For this review, take the finished solid that the model builds, in its own axes (mm). A direction names the side the tool comes from. Coordinates: 2 decimals unless noted, no trailing zeros. Loops run counter-clockwise (first coordinate to the right, second up) from the corner with the lowest first, then second, coordinate; pieces in that order, holes last. Notation, with made-up numbers: M 85,75.5 L 99,75.5 A28 cw 99,94.5 Z; hole C -39,-10.75 d11. An arc over 180 degrees is marked long. Put each result on its own line as item: value.
Autodesk Fusion 360 part; units mm, degrees
sketch "Sketch1" plane through (0, 0, 0) normal (0, 0, 1) x (1, 0, 0)
  line L0 (21.15, -21.15) -> (-21.15, -21.15)
  line L1 (-21.15, -21.15) -> (-21.15, 21.15)
  line L2 (-21.15, 21.15) -> (21.15, 21.15)
  line L3 (21.15, 21.15) -> (21.15, -21.15)
  line L4 (21.15, -21.15) -> (-21.15, 21.15) construction
  line L5 (-21.15, -21.15) -> (21.15, 21.15) construction
  dimension "d3" = 42.3
  dimension "d4" = 42.3
extrude "Extrude1" add sketch "Sketch1" along normal blind 39
chamfer "Chamfer1" distance 6 angle 45 4 edges at (-21.15, 0, 39) (21.15, 0, 39) (21.15, 0, 0) (-21.15, 0, 0)
sketch "Sketch2" plane through (0, -21.15, 0) normal (0, -1, 0) x (1, 0, 0)
  line L0 (-21.15, 6) -> (-15.15, 0)
  line L1 (-15.15, 0) -> (15.15, 0)
  line L2 (15.15, 0) -> (21.15, 6)
  line L3 (21.15, 6) -> (21.15, 33)
  line L4 (21.15, 33) -> (15.15, 39)
  line L5 (15.15, 39) -> (-15.15, 39)
  line L6 (-15.15, 39) -> (-21.15, 33)
  line L7 (-21.15, 33) -> (-21.15, 6)
  circle A0 centre (0, 20) radius 2.5
  dimension "d8" = 5
extrude "Extrude2" add sketch "Sketch2" along normal blind 21 contours A0
sketch "Sketch3" plane through (0, -21.15, 0) normal (0, -1, 0) x (1, 0, 0)
  circle A0 centre (0, 20) radius 2.5
  line L0 (-21.15, 6) -> (-15.15, 0)
  line L1 (-15.15, 0) -> (15.15, 0)
  line L2 (15.15, 0) -> (21.15, 6)
  line L3 (21.15, 6) -> (21.15, 33)
  line L4 (21.15, 33) -> (15.15, 39)
  line L5 (15.15, 39) -> (-15.15, 39)
  line L6 (-15.15, 39) -> (-21.15, 33)
  line L7 (-21.15, 33) -> (-21.15, 6)
  circle A1 centre (0, 20) radius 11
  dimension "d11" = 22
extrude "Extrude3" add sketch "Sketch3" along normal blind 2 contours A1
sketch "Sketch4" plane through (0, -21.15, 0) normal (0, -1, 0) x (1, 0, 0)
  circle A0 centre (0, 20) radius 11
  line L0 (-21.15, 6) -> (-15.15, 0)
  line L1 (-15.15, 0) -> (15.15, 0)
  line L2 (15.15, 0) -> (21.15, 6)
  line L3 (21.15, 6) -> (21.15, 33)
  line L4 (21.15, 33) -> (15.15, 39)
  line L5 (15.15, 39) -> (-15.15, 39)
  line L6 (-15.15, 39) -> (-21.15, 33)
  line L7 (-21.15, 33) -> (-21.15, 6)
  circle A1 centre (-15.0778, 34.9879) radius 1.5
  circle A2 centre (15.0778, 5.0121) radius 1.5
  circle A3 centre (14.9957, 34.9599) radius 1.5
  circle A4 centre (-15.1592, 5.2464) radius 1.5
  dimension "d14" = 3
  dimension "d16" = 360
  dimension "d17" = 3
  dimension "d18" = 3
extrude "Extrude4" cut sketch "Sketch4" against normal blind 4.5 contours A1 | A2 | A3 | A4
sketch "Sketch5" plane through (0, 21.15, 0) normal (0, 1, 0) x (-1, 0, 0)
  line L0 (15.15, 0) -> (21.15, 6)
  line L1 (21.15, 6) -> (21.15, 33)
  line L2 (21.15, 33) -> (15.15, 39)
  line L3 (15.15, 39) -> (-15.15, 39)
  line L4 (-15.15, 39) -> (-21.15, 33)
  line L5 (-21.15, 33) -> (-21.15, 6)
  line L6 (-21.15, 6) -> (-15.15, 0)
  line L7 (-15.15, 0) -> (15.15, 0)
  line L8 (-11.15, 39) -> (-21.15, 29)
  line L9 (-21.15, 29) -> (-21.15, 39)
  line L10 (-11.15, 39) -> (-21.15, 39)
  dimension "d21" = 10
  dimension "d22" = 10
extrude "Extrude5" cut sketch "Sketch5" against normal blind 22 from surface at -8 contours L3 L4 L5 L8 L9 L10 | L4 L9 L10
sketch "Sketch6" plane through (0, 21.15, 0) normal (0, 1, 0) x (-1, 0, 0)
  line L0 (15.15, 0) -> (21.15, 6)
  line L1 (21.15, 6) -> (21.15, 33)
  line L2 (21.15, 33) -> (15.15, 39)
  line L3 (15.15, 39) -> (-15.15, 39)
  line L4 (-15.15, 39) -> (-21.15, 33)
  line L5 (-21.15, 33) -> (-21.15, 6)
  line L6 (-21.15, 6) -> (-15.15, 0)
  line L7 (-15.15, 0) -> (15.15, 0)
  line L8 (11.15, 39) -> (21.15, 29)
  line L9 (11.15, 39) -> (21.15, 39)
  line L10 (21.15, 29) -> (21.15, 39)
  dimension "d26" = 10
  dimension "d27" = 10
extrude "Extrude6" cut sketch "Sketch6" against normal blind 22 from surface at -8 contours L1 L2 L3 L8 L9 L10 | L2 L9 L10
sketch "Sketch7" plane through (0, 21.15, 0) normal (0, 1, 0) x (-1, 0, 0)
  line L0 (15.15, 0) -> (21.15, 6)
  line L1 (21.15, 6) -> (21.15, 33)
  line L2 (21.15, 33) -> (15.15, 39)
  line L3 (15.15, 39) -> (-15.15, 39)
  line L4 (-15.15, 39) -> (-21.15, 33)
  line L5 (-21.15, 33) -> (-21.15, 6)
  line L6 (-21.15, 6) -> (-15.15, 0)
  line L7 (-15.15, 0) -> (15.15, 0)
  line L8 (21.15, 10) -> (11.15, 0)
  line L9 (11.15, 0) -> (21.15, 0)
  line L10 (21.15, 10) -> (21.15, 0)
  dimension "d31" = 10
  dimension "d32" = 10
extrude "Extrude7" cut sketch "Sketch7" against normal blind 22 from surface at -8 contours L0 L1 L7 L8 L9 L10 | L0 L9 L10
sketch "Sketch8" plane through (0, 21.15, 0) normal (0, 1, 0) x (-1, 0, 0)
  line L0 (15.15, 0) -> (21.15, 6)
  line L1 (21.15, 6) -> (21.15, 33)
  line L2 (21.15, 33) -> (15.15, 39)
  line L3 (15.15, 39) -> (-15.15, 39)
  line L4 (-15.15, 39) -> (-21.15, 33)
  line L5 (-21.15, 33) -> (-21.15, 6)
  line L6 (-21.15, 6) -> (-15.15, 0)
  line L7 (-15.15, 0) -> (15.15, 0)
  line L8 (-11.15, 0) -> (-21.15, 10)
  line L9 (-11.15, 0) -> (-21.15, 0)
  line L10 (-21.15, 10) -> (-21.15, 0)
  dimension "d36" = 10
  dimension "d37" = 10
extrude "Extrude8" cut sketch "Sketch8" against normal blind 22 from surface at -8 contours L5 L6 L7 L8 L9 L10 | L6 L9 L10
sketch "Sketch9" plane through (0, 13.15, 0) normal (0, -1, 0) x (1, 0, 0)
  line L0 (21.15, 33) -> (15.15, 39)
  line L1 (15.15, 39) -> (11.15, 39)
  line L2 (21.15, 29) -> (21.15, 33)
sketch "Sketch10" plane through (0, 13.15, 0) normal (0, -1, 0) x (1, 0, 0)
sketch "Sketch11" plane through (0, 13.15, 0) normal (0, -1, 0) x (1, 0, 0)
sketch "Sketch12" plane through (0, 13.15, 0) normal (0, -1, 0) x (1, 0, 0)
(1) Add section C-C (y = 5.5). Write out the cut boundary in (x, z), plus the area to 3 significant figures.
Determined:
outline: M -21.15,10 L -11.15,0 L 11.15,0 L 21.15,10 L 21.15,29 L 11.15,39 L -11.15,39 L -21.15,29 Z
area: 1,450 mm^2
(2) Wall thickness on line 1 along Y through (x, z) = (18, 7.5); line 2 along Y through (x, z) = (-14.5, 6); line 3 along X through (y, z) = (-25.5, 20.5): over which ranges is each line inside the solid? List them lowest first. Write a range as [from, to].
Determined:
line 1: y = [-21.15, 21.15]
line 2: y = [-16.65, 21.15]
line 3: x = [-2.45, 2.45]
(3) Add section B-B (z = 20). Write out the cut boundary in (x, y), plus the area to 3 significant figures.
Determined:
outline: M -21.15,-21.15 L -11,-21.15 L -11,-23.15 L -2.5,-23.15 L -2.5,-42.15 L 2.5,-42.15 L 2.5,-23.15 L 11,-23.15 L 11,-21.15 L 21.15,-21.15 L 21.15,21.15 L -21.15,21.15 Z
area: 1,930 mm^2
(4) Draft analysis for pull direction Z (two halves, no side actions). For faces 1 (the flat face through (15, -16.65, 35)), 2 (the flat face through (16.08, 2.3, 4.93)), 3 (the flat face through (0, -42.15, 20)), state which applies: +Z half, -Z half, draft (parallel to the pull), parting line (faces both ways), or undercut.
Determined:
face 1: undercut
face 2: -Z half
face 3: draft
(5) Add section A-A (x = -12.5). Write out the cut boundary in (y, z).
Determined:
outline: M -21.15,0 L -8.85,0 L -8.85,1.35 L 13.15,1.35 L 13.15,0 L 21.15,0 L 21.15,39 L 13.15,39 L 13.15,37.65 L -8.85,37.65 L -8.85,39 L -21.15,39 Z
(6) For pin 1 (2.5 mm diameter, centred on x = 15, z = 5.5, fed in from -Y); pin 2 (8 mm diameter, centred on y = -33, z = 22, fed in from -X); pin 3 (2.5 mm diameter, centred on x = 15.08, z = 5.01, fed in from -Y); pin 4 (6 mm diameter, centred on x = -7, y = -31.5, fed in from +Z), all flat-tipped, find the tip position at first contact; note any pin that passes through.
Determined:
pin 1: stops at y = -21.15
pin 2: stops at x = -2.5
pin 3: stops at y = -16.65
pin 4: passes through
(7) Add section D-D (y = -32.5). Write out the cut boundary in (x, z), plus the area to 3 significant figures.
Determined:
outline: C 0,20 d5
area: 19.6 mm^2
(8) Tool access review of faces 4 (the flat face through (-17, 13.15, 35)), 5 (the flat face through (16.08, 2.3, 34.07)), 6 (the flat face through (15, -16.65, 5)): name each direction out of +Z, -Z, +X, -X, +Y, -Y from which nothing blocks a thin tool from reaching the whole face with its end or side.
Determined:
face 4: +Z, -X
face 5: +Z, +X
face 6: -Y
